Source: CAD feature listing. Evaluate the final solid. Frame: model axes, mm. A direction names the side the tool comes from. Round coordinates to 2 decimals unless told otherwise and drop trailing zeros. Order: outer loops, then holes, each group sorted by start corner. A loop starts at its lowest first (then second) coordinate and runs counter-clockwise, first axis right, second up. Notation, with made-up numbers: (-23, 76.25) -> (-18, 76.25) arc R17 ccw to (-18, 97.25) -> close; hole circle Ø7 at (-25, 70.5). An arc over 180 degrees is marked (long way). Use a Markdown table: item, result. Add a question column.
Autodesk Inventor part; units mm, degrees
ref_plane "YZ Plane" through (0, 0, 0) normal (1, 0, 0) x (0, 1, 0)
ref_plane "XZ Plane" through (0, 0, 0) normal (0, 1, 0) x (-1, 0, 0)
ref_plane "XY Plane" through (0, 0, 0) normal (0, 0, 1) x (1, 0, 0)
sketch "Эскиз1" plane through (0, 0, 0) normal (0, 1, 0) x (-1, 0, 0)
  line L0 (-50, 75) -> (50, 75)
  line L1 (50, 75) -> (50, -75)
  line L2 (50, -75) -> (-50, -75)
  line L3 (-50, -75) -> (-50, 75)
  line L4 (-50, 75) -> (50, -75) construction
  line L5 (50, 75) -> (-50, -75) construction
  point P0 (0, 0)
  dimension "d0" = 150
  dimension "d1" = 100
extrude "Выдавливание1" add sketch "Эскиз1" along normal blind 4
sketch "Эскиз2" plane through (0, 4, 0) normal (0, 1, 0) x (1, 0, 0)
  line L0 (50, 75) -> (-50, 75)
  line L1 (50, -75) -> (-50, -75)
  line L2 (-50, -75) -> (-50, 75)
  line L3 (-50, 75) -> (50, 75)
  line L4 (50, 75) -> (50, -75)
  line L5 (50, -75) -> (-50, 75) construction
  line L6 (-50, -75) -> (50, 75) construction
  line L7 (46, -71) -> (-46, -71)
  line L8 (-46, -71) -> (-46, 71)
  line L9 (-46, 71) -> (46, 71)
  line L10 (46, 71) -> (46, -71)
  line L11 (46, -71) -> (-46, 71) construction
  line L12 (-46, -71) -> (46, 71) construction
  point P0 (0, 0)
  dimension "d4" = 4
  dimension "d5" = 4
extrude "Выдавливание2" add sketch "Эскиз2" along normal blind 60
sketch "Эскиз3" plane through (50, 0, 75) normal (1, 0, 0) x (0, 0, -1)
  line L0 (150, 0) -> (0, 0)
  circle A0 centre (15, 20) radius 2
  point P0 (75, 0)
  dimension "d10" = 4
extrude "Выдавливание3" cut sketch "Эскиз3" against normal blind 135.5
sketch "Эскиз4" plane through (50, 0, 75) normal (1, 0, 0) x (0, 0, -1)
  line L0 (150, 0) -> (0, 0)
  line L1 (146, 4) -> (4, 4)
  line L2 (135, 4) -> (105, 4)
  line L3 (105, 4) -> (105, 27)
  line L4 (105, 27) -> (135, 27)
  line L5 (135, 27) -> (135, 4)
  point P0 (75, 0)
  dimension "d14" = 23
  dimension "d15" = 30
extrude "Выдавливание4" cut sketch "Эскиз4" against normal blind 135.5
properties part number "эвакуатор"
1) Reachability of faces 1 (the flat face through (-1, 34, -71)), 2 (the flat face through (1, 0, 1)), 3 (the flat face through (48, 16, -60)) from +Z, -Z, +X, -X, +Y, -Y: full face, straight path, thin tool, end or side. Return the list, or none.
2) Section D-D on x = -14.5. Output: boundary loops of the cut face in (y, z), then the cut area to 3 significant figures.
3) Line query: probe 1 along X at (y, z) = (57.5, 13.5); probe 2 along Z at (x, y) = (28.5, 9); probe 3 along Y at (x, z) = (47.65, 60). Output: solid intervals per line, ascending. Write a range as from..to.
4) Section C-C on y = 56. Output: boundary loops of the cut face in (x, z).
5) Section A-A on z = 60. Output: boundary loops of the cut face in (x, y), then the cut area to 3 significant figures.
6) Section B-B on y = 20. Output: boundary loops of the cut face in (x, z), then the cut area to 3 significant figures.
7) Draft query along Y for faces 4 (the flat face through (-48, 64, 0)), 5 (the flat face through (-1, 32, -75)), 6 (the flat face through (48, 27, -45)), 7 (the flat face through (-48, 27, -45)). Return one class per face: pulls with the +Y half, pulls with the -Y half, needs draft (parallel to the pull), parting line crosses it, or undercut.
Conclusion:
| question | item | result |
|---|---|---|
| 1 | face 1 | +Y |
| 1 | face 2 | +Z, -Z, +X, -X, -Y |
| 1 | face 3 | +X, -X |
| 2 | outline | (0, -75) -> (64, -75) -> (64, -71) -> (4, -71) -> (4, 71) -> (64, 71) -> (64, 75) -> (0, 75) -> close |
| 2 | area | 1,080 mm^2 |
| 3 | probe 1 | x = -50..-46, 46..50 |
| 3 | probe 2 | z = -75..-71, 71..75 |
| 3 | probe 3 | y = 0..18, 22..64 |
| 4 | outline | (-50, -75) -> (50, -75) -> (50, 75) -> (-50, 75) -> close; hole (-46, -71) -> (46, -71) -> (46, 71) -> (-46, 71) -> close |
| 5 | outline | (-50, 0) -> (50, 0) -> (50, 18) -> (46, 18) -> (46, 4) -> (-46, 4) -> (-46, 18) -> (-50, 18) -> close; (-50, 22) -> (-46, 22) -> (-46, 64) -> (-50, 64) -> close; (46, 22) -> (50, 22) -> (50, 64) -> (46, 64) -> close |
| 5 | area | 848 mm^2 |
| 6 | outline | (-50, -75) -> (50, -75) -> (50, -60) -> (46, -60) -> (46, -71) -> (-46, -71) -> (-46, -60) -> (-50, -60) -> close; (-50, -30) -> (-46, -30) -> (-46, 58) -> (-50, 58) -> close; (-50, 62) -> (-46, 62) -> (-46, 71) -> (46, 71) -> (46, 62) -> (50, 62) -> (50, 75) -> (-50, 75) -> close; (46, -30) -> (50, -30) -> (50, 58) -> (46, 58) -> close |
| 6 | area | 1,660 mm^2 |
| 7 | face 4 | pulls with the +Y half |
| 7 | face 5 | needs draft |
| 7 | face 6 | undercut |
| 7 | face 7 | undercut |
